For this review, take the finished solid that the model builds, in its own axes (mm). Give positions to 0.01 mm unless a question says otherwise; leave off trailing zeros. Loops run counter-clockwise (first coordinate to the right, second up) from the corner with the lowest first, then second, coordinate; pieces in that order, holes last. Notation, with made-up numbers: (41.25, -15.75) -> (70.25, -15.75) arc R16 ccw to (70.25, 4.25) -> close; hole circle Ø2 at (15.5, -4.5). An arc over 180 degrees is marked (long way). One line per question, with ' | ' between items. Start each with the question number.
(1) Insertion check: P1, Ø1.5, axis at y = -4, z = 1.5, coming from the -X side; P2, Ø1, axis at x = -1, y = -18, coming from the -Z side. Each pin has a flat end and moves straight along its axis. Give the tip position at first contact, or say it passes through.
(2) Consider section A-A (y = -7). Write out the cut boundary in (x, z).
(3) Wall thickness on probe 1 along X at (y, z) = (-4, 0.1); probe 2 along Z at (x, y) = (-0.75, -28.5): over which ranges is each line inside the solid? List them lowest first.
(4) Consider section B-B (y = -30.5). Write out the cut boundary in (x, z), and give its area (3 significant figures).
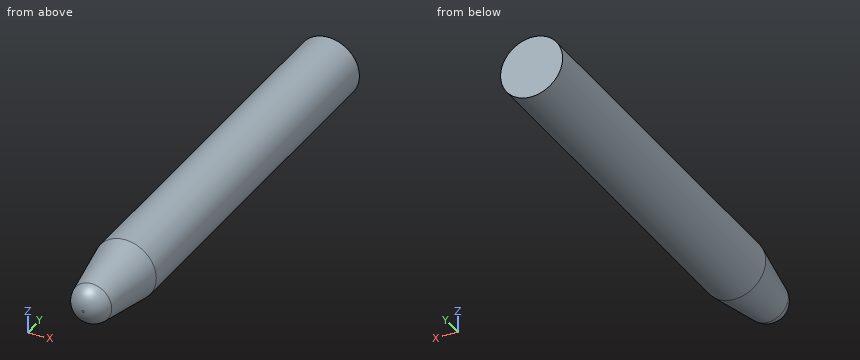
from build123d import *

# Parameters (mm, degrees)
F0_R     = 2.25
F1_DEPTH = 33
F2_SIZE2 = 1
F2_SIZE  = 5.6712818196
F3_R     = 1.4


with BuildPart() as f1:
    # F0 (on Front) → F1 (new body)
    with BuildSketch(Plane.XZ):
        Circle(F0_R)
    extrude(amount=F1_DEPTH)

    # F2
    f2_edges = [f1.edges().sort_by_distance(p)[0] for p in [
        (-2.25, -33, 0),
    ]]
    f2_side = f1.faces().sort_by_distance((-2.25, -16.5, 0))[0]
    chamfer(f2_edges, length=F2_SIZE, length2=F2_SIZE2, reference=f2_side)

    # F3
    f3_edges = [f1.edges().sort_by_distance(p)[0] for p in [
        (-1.25, -33, 0),
    ]]
    fillet(f3_edges, radius=F3_R)


solid = f1.part
A:
1) P1: stops at x = -2.12 | P2: stops at z = -2.19
2) outline: circle Ø4.5 at (0, 0)
3) probe 1: x = -2.25 to 2.25 | probe 2: z = -1.9 to 1.9
4) outline: circle Ø3.38 at (0, 0) | area: 8.98 mm^2
